Geometry check sheet. Reference: the model listing, model coordinates, mm. A direction names the side the tool comes from. Round coordinates to 2 decimals unless told otherwise and drop trailing zeros. Order: outer loops, then holes, each group sorted by start corner. A loop starts at its lowest first (then second) coordinate and runs counter-clockwise, first axis right, second up. Notation, with made-up numbers: (61.5, 11) -> (78.5, 11) arc R29 ccw to (78.5, 31) -> close; hole circle Ø11 at (-25, -15). An arc over 180 degrees is marked (long way). Use a Markdown table: item, result. Add a question column.
Item 1: Sectioned sample at C-C, the plane z = -38. Record the cut outline in (x, y) (1 decimal), and give its area (3 significant figures).
Item 2: Sectioned sample at D-D, the plane z = -11.5. Record the cut outline in (x, y) (1 decimal).
Item 3: Gauge pin test, flat ends, axial feed: pin 1 Ø4.5 at (x, y) = (-68.26, 38.1) entering from +Z; pin 2 Ø3.5 at (x, y) = (-68.26, 0) entering from +Z; pin 3 Ø6 at (x, y) = (-28, -24.5) entering from +Z. Record the tip position at first contact, or that the pin passes through.
Item 4: Sectioned sample at B-B, the plane y = 28. Record the cut outline in (x, z) (3 decimals), and give its area (3 significant figures).
Item 5: Sectioned sample at A-A, the plane z = -25. Record the cut outline in (x, y) (1 decimal).
Item 6: Material ranges on probe 1 along Y at (x, z) = (34, -33); probe 2 along X at (y, z) = (19.5, -6) (3 decimals); probe 3 along X at (y, z) = (-38, -19) (3 decimals), recorded low to high. Write a range as [from, to].
Item 7: Mould release check, pull along Y, two halves, no side actions. Record for faces 3 (the conical face through (67.776, 38.121, -21.39)), 4 (the flat face through (-1, -52.388, -25)), 5 (the cylindrical face through (-48.065, 50.968, -25.766)): pulls with the +Y half, pulls with the -Y half, needs draft (parallel to the pull), parting line crosses it, or undercut.
Item 8: Set-up check for faces 1 (the cylindrical face through (-48.065, -51.007, -25.766)), 2 (the cylindrical face through (68.627, -35.323, -10.14)): record each of +Z, -Z, +X, -X, +Y, -Y from which the full face is reachable in a straight line by a thin tool's end or side.
from build123d import *

# Parameters (mm, degrees)
F0_W     = 5
F0_H     = 104.775
F0_W_2   = 146.05
F0_R     = 3.24
F1_DEPTH = 50
F2_W     = 119.824
F2_H     = 99.175
F3_DEPTH = 45
F4_D     = 5.6
F4_DEPTH = 20
F4_TIP   = 1.6824097333
F5_W     = 40
F5_H     = 5
F6_DEPTH = 104.776
F7_D     = 4


with BuildPart() as f1:
    # F0 (on Top) → F1 (new body)
    with BuildSketch(Plane.XY):
        with Locations((-75.525, 0)):
            Rectangle(F0_W, F0_H)
        Rectangle(F0_W_2, F0_H)
        with Locations((-68.262, -38.0995)):
            Circle(F0_R, mode=Mode.SUBTRACT)
        with Locations((68.262, -38.0995)):
            Circle(F0_R, mode=Mode.SUBTRACT)
        with Locations((-68.262, 0.0005)):
            Circle(F0_R, mode=Mode.SUBTRACT)
        with BuildLine():
            ThreePointArc((68.262, 44.4495), (61.912, 38.0995), (68.262, 31.7495))
            Line((68.262, 31.7495), (72.225, 31.7495))
            Line((72.225, 31.7495), (72.225, 6.3505))
            Line((72.225, 6.3505), (68.262, 6.3505))
            ThreePointArc((68.262, 6.3505), (61.912, 0.0005), (68.262, -6.3495))
            Line((68.262, -6.3495), (72.225, -6.3495))
            Line((72.225, -6.3495), (72.225, -31.7495))
            Line((72.225, -31.7495), (68.262, -31.7495))
            ThreePointArc((68.262, -31.7495), (61.912, -38.0995), (68.262, -44.4495))
            Line((68.262, -44.4495), (72.225, -44.4495))
            Line((72.225, -44.4495), (72.225, -51.5875))
            Line((72.225, -51.5875), (-72.225, -51.5875))
            Line((-72.225, -51.5875), (-72.225, -44.4495))
            Line((-72.225, -44.4495), (-68.262, -44.4495))
            ThreePointArc((-68.262, -44.4495), (-61.912, -38.0995), (-68.262, -31.7495))
            Line((-68.262, -31.7495), (-72.225, -31.7495))
            Line((-72.225, -31.7495), (-72.225, -6.3495))
            Line((-72.225, -6.3495), (-68.262, -6.3495))
            ThreePointArc((-68.262, -6.3495), (-61.912, 0.0005), (-68.262, 6.3505))
            Line((-68.262, 6.3505), (-72.225, 6.3505))
            Line((-72.225, 6.3505), (-72.225, 31.7495))
            Line((-72.225, 31.7495), (-68.262, 31.7495))
            ThreePointArc((-68.262, 31.7495), (-61.912, 38.0995), (-68.262, 44.4495))
            Line((-68.262, 44.4495), (-72.225, 44.4495))
            Line((-72.225, 44.4495), (-72.225, 51.5875))
            Line((-72.225, 51.5875), (72.225, 51.5875))
            Line((72.225, 51.5875), (72.225, 44.4495))
            Line((72.225, 44.4495), (68.262, 44.4495))
        make_face(mode=Mode.SUBTRACT)
        with Locations((-68.262, 38.0995)):
            Circle(F0_R, mode=Mode.SUBTRACT)
        with Locations((68.262, 0.0005)):
            Circle(F0_R, mode=Mode.SUBTRACT)
        with Locations((68.262, 38.0995)):
            Circle(F0_R, mode=Mode.SUBTRACT)
        with Locations((75.525, 0)):
            Rectangle(F0_W, F0_H)
        with Locations((-68.262, 38.0995)):
            Circle(F0_R)
        with BuildLine():
            Line((72.225, 31.7495), (68.262, 31.7495))
            ThreePointArc((68.262, 31.7495), (61.912, 38.0995), (68.262, 44.4495))
            Line((68.262, 44.4495), (72.225, 44.4495))
            Line((72.225, 44.4495), (72.225, 51.5875))
            Line((72.225, 51.5875), (-72.225, 51.5875))
            Line((-72.225, 51.5875), (-72.225, 44.4495))
            Line((-72.225, 44.4495), (-68.262, 44.4495))
            ThreePointArc((-68.262, 44.4495), (-61.912, 38.0995), (-68.262, 31.7495))
            Line((-68.262, 31.7495), (-72.225, 31.7495))
            Line((-72.225, 31.7495), (-72.225, 6.3505))
            Line((-72.225, 6.3505), (-68.262, 6.3505))
            ThreePointArc((-68.262, 6.3505), (-61.912, 0.0005), (-68.262, -6.3495))
            Line((-68.262, -6.3495), (-72.225, -6.3495))
            Line((-72.225, -6.3495), (-72.225, -31.7495))
            Line((-72.225, -31.7495), (-68.262, -31.7495))
            ThreePointArc((-68.262, -31.7495), (-61.912, -38.0995), (-68.262, -44.4495))
            Line((-68.262, -44.4495), (-72.225, -44.4495))
            Line((-72.225, -44.4495), (-72.225, -51.5875))
            Line((-72.225, -51.5875), (72.225, -51.5875))
            Line((72.225, -51.5875), (72.225, -44.4495))
            Line((72.225, -44.4495), (68.262, -44.4495))
            ThreePointArc((68.262, -44.4495), (61.912, -38.0995), (68.262, -31.7495))
            Line((68.262, -31.7495), (72.225, -31.7495))
            Line((72.225, -31.7495), (72.225, -6.3495))
            Line((72.225, -6.3495), (68.262, -6.3495))
            ThreePointArc((68.262, -6.3495), (61.912, 0.0005), (68.262, 6.3505))
            Line((68.262, 6.3505), (72.225, 6.3505))
            Line((72.225, 6.3505), (72.225, 31.7495))
        make_face()
        with Locations((-68.262, 0.0005)):
            Circle(F0_R)
        with Locations((-68.262, -38.0995)):
            Circle(F0_R)
        with Locations((68.262, -38.0995)):
            Circle(F0_R)
        with Locations((68.262, 0.0005)):
            Circle(F0_R)
        with Locations((68.262, 38.0995)):
            Circle(F0_R)
    extrude(amount=-F1_DEPTH)

    # F2 (on face) → F3 (cut)
    with BuildSketch(Plane.XY):
        Rectangle(F2_W, F2_H)
    extrude(amount=-F3_DEPTH, mode=Mode.SUBTRACT)

    # F4
    with Locations(Plane.XY):
        with Locations((-68.262, 38.0995), (-68.262, 0.0005), (-68.262, -38.0995), (68.262, -38.0995), (68.262, 38.0995), (68.262, 0.0005)):
            Hole(F4_D / 2, depth=F4_DEPTH)
            with Locations((0, 0, -(F4_DEPTH + F4_TIP / 2))):  # 118° drill point
                Cone(0, F4_D / 2, F4_TIP, mode=Mode.SUBTRACT)

    # F5 (on face) → F6 (cut, through all)
    with BuildSketch(Plane(origin=(0, 52.3875, 0), x_dir=(-1, 0, 0), z_dir=(0, 1, 0))):
        with Locations((0, -42.5)):
            Rectangle(F5_W, F5_H)
    extrude(amount=-F6_DEPTH, mode=Mode.SUBTRACT)

    # F7 (through all)
    with Locations(Plane(origin=(0, 52.3875, 0), x_dir=(-1, 0, 0), z_dir=(0, 1, 0))):
        with Locations((-49.912, -25), (49.912, -25)):
            Hole(F7_D / 2)


solid = f1.part
Found:
| question | item | result |
|---|---|---|
| 1 | outline | (-78, -52.4) -> (78, -52.4) -> (78, 52.4) -> (-78, 52.4) -> close; hole (-59.9, -49.6) -> (59.9, -49.6) -> (59.9, 49.6) -> (-59.9, 49.6) -> close |
| 1 | area | 4,470 mm2 |
| 2 | outline | (-78, -52.4) -> (78, -52.4) -> (78, 52.4) -> (-78, 52.4) -> close; hole circle Ø5.6 at (-68.3, -38.1); hole circle Ø5.6 at (-68.3, 0); hole circle Ø5.6 at (-68.3, 38.1); hole (-59.9, -49.6) -> (59.9, -49.6) -> (59.9, 49.6) -> (-59.9, 49.6) -> close; hole circle Ø5.6 at (68.3, -38.1); hole circle Ø5.6 at (68.3, 0); hole circle Ø5.6 at (68.3, 38.1) |
| 3 | pin 1 | stops at z = -20.33 |
| 3 | pin 2 | stops at z = -20.63 |
| 3 | pin 3 | stops at z = -45 |
| 4 | outline | (-78.025, -50) -> (78.025, -50) -> (78.025, 0) -> (59.912, 0) -> (59.912, -45) -> (-59.912, -45) -> (-59.912, 0) -> (-78.025, 0) -> close |
| 4 | area | 2,410 mm2 |
| 5 | outline | (-78, -52.4) -> (-51.9, -52.4) -> (-51.9, -49.6) -> (-59.9, -49.6) -> (-59.9, 49.6) -> (-51.9, 49.6) -> (-51.9, 52.4) -> (-78, 52.4) -> close; (-47.9, -52.4) -> (47.9, -52.4) -> (47.9, -49.6) -> (-47.9, -49.6) -> close; (-47.9, 49.6) -> (47.9, 49.6) -> (47.9, 52.4) -> (-47.9, 52.4) -> close; (51.9, -52.4) -> (78, -52.4) -> (78, 52.4) -> (51.9, 52.4) -> (51.9, 49.6) -> (59.9, 49.6) -> (59.9, -49.6) -> (51.9, -49.6) -> close |
| 6 | probe 1 | y = [-52.39, -49.59], [49.59, 52.39] |
| 6 | probe 2 | x = [-78.025, -59.912], [59.912, 78.025] |
| 6 | probe 3 | x = [-78.025, -71.06], [-65.464, -59.912], [59.912, 65.464], [71.06, 78.025] |
| 7 | face 3 | undercut |
| 7 | face 4 | pulls with the -Y half |
| 7 | face 5 | needs draft |
| 8 | face 1 | +Y, -Y |
| 8 | face 2 | +Z |
